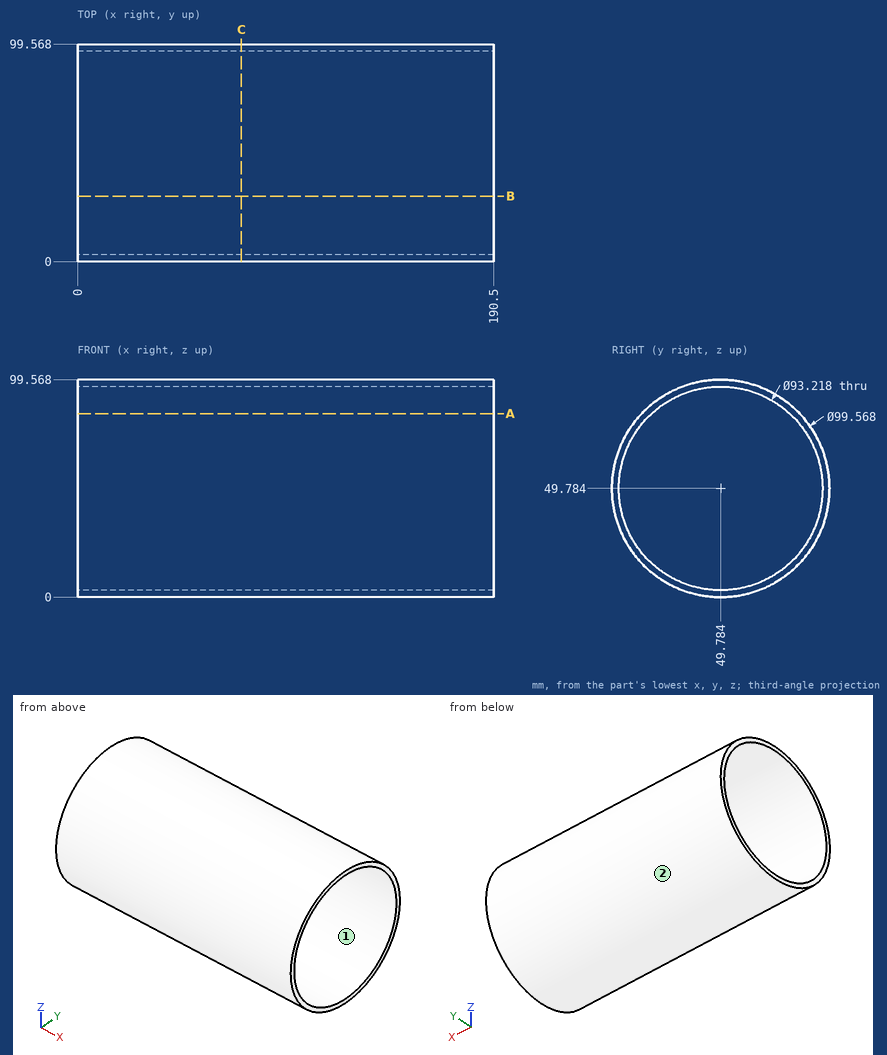
Answer from the drawing. Dimensions are ordinates in mm from the lowest x, y and z of the part. Coordinates: 2 decimals unless noted, no trailing zeros. Write each loop counter-clockwise with the first axis right and the second up, starting at its lowest first coordinate (ties: lowest second). Pieces come first, ordered by that corner, then holes. Notation, with made-up numbers: M 80,-34 L 105,-34 A19 cw 105,-6 Z; hole C -29.5,51.25 d11. An arc over 180 degrees is marked long. Write item = value, one per line.
1. The part is cut by section A-A (z = 84). Determine the outline of the cut face in (x, y), then the cut area to 3 significant figures.
Solution:
outline = M 0,13.62 L 190.5,13.62 L 190.5,18.13 L 0,18.13 Z; M 0,81.43 L 190.5,81.43 L 190.5,85.95 L 0,85.95 Z
area = 1,720 mm2
2. Determine the mould class of the marked faces 1 and 2 for opening direction Z: released by +Z, released by -Z, zero draft, split by the parting line, or undercut.
Solution:
face_1 = undercut
face_2 = split by the parting line
3. The part is cut by section C-C (x = 75). Determine the outline of the cut face in (y, z), then the cut area to 3 significant figures.
Solution:
outline = C 49.78,49.78 d99.57; hole C 49.78,49.78 d93.22
area = 961 mm2
4. Flat-ended cylindrical pins translate along their axes: pin 1 (5 mm diameter, centred on y = 82.5, z = 23.5, fed in from -X); pin 2 (6 mm diameter, centred on x = 53.5, y = 66.5, fed in from +Z); pin 3 (3 mm diameter, centred on x = 43, y = 24.5, fed in from +Z); pin 4 (2 mm diameter, centred on x = 133.5, y = 11.5, fed in from +Z). Find the tip coordinate at first contact, or state that the pin passes through.
Solution:
pin_1 = through
pin_2 = 97.64
pin_3 = 93.52
pin_4 = 82.77
5. Straight lines are drawn through the part: line 1 (Y direction, x = 12.5, z = 84.5); line 2 (Z direction, x = 112.5, y = 69.5); line 3 (Y direction, x = 91, z = 32). For each, find the intervals that lie inside material, in ascending order. Write a range as from..to.
Solution:
line_1 = 14.1..18.68, 80.88..85.47
line_2 = 4.07..7.55, 92.02..95.5
line_3 = 3.28..6.7, 92.87..96.28
6. The part is cut by section B-B (y = 30). Determine the outline of the cut face in (x, z).
Solution:
outline = M 0,4.1 L 190.5,4.1 L 190.5,7.58 L 0,7.58 Z; M 0,91.99 L 190.5,91.99 L 190.5,95.47 L 0,95.47 Z
